Verification items for this drawing (mm, ordinates from the low corner). Round coordinates to 2 decimals unless told otherwise and drop trailing zeros. Loops run counter-clockwise (first coordinate to the right, second up) from the corner with the lowest first, then second, coordinate; pieces in that order, holes last. Notation, with made-up numbers: (-9.75, 46) - (43.25, 46) arc R12 cw to (43.25, 53) - close; hole circle Ø10 at (15.25, 78.5). An arc over 180 degrees is marked (long way). Put each result on its own line as item: value.
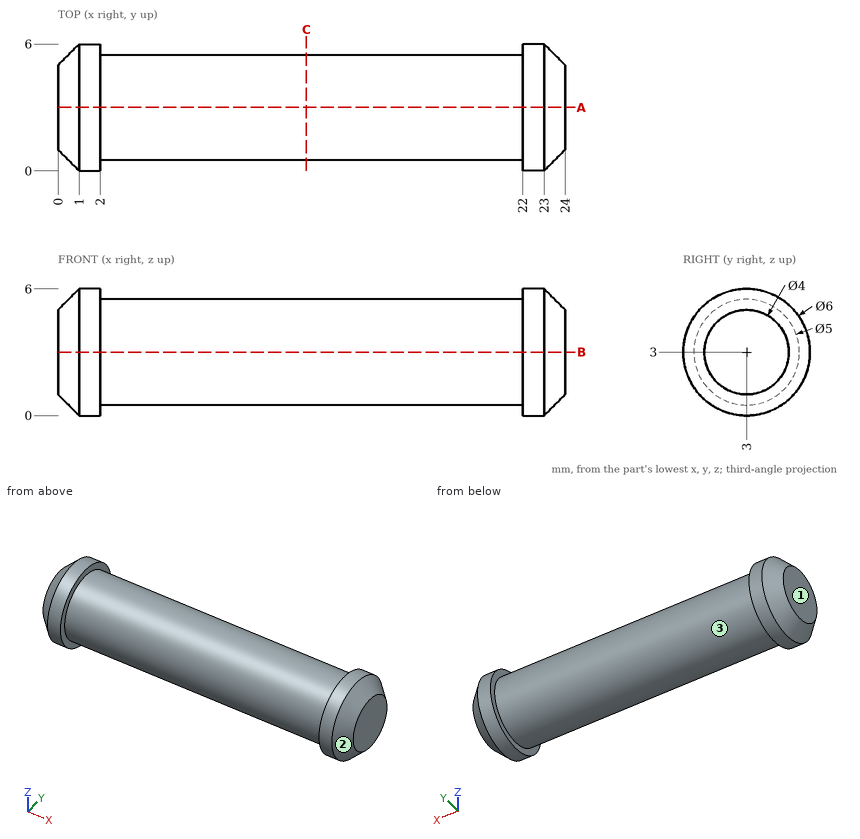
Item 1: Go/stop test with flat-tipped pins: pin 1 (1.5 mm diameter, centred on x = 4, y = 4.5, fed in from +Z); pin 2 (2 mm diameter, centred on x = 10.5, y = 1.5, fed in from -Z). Record where each tip stops, or that it passes through.
Filled sheet:
pin 1: z = 5.38
pin 2: z = 0.55
Item 2: Section check A-A on y = 3. Enter the section's corners in (x, z).
Filled sheet:
outline: (0, 1) - (1, 0) - (2, 0) - (2, 0.5) - (22, 0.5) - (22, 0) - (23, 0) - (24, 1) - (24, 5) - (23, 6) - (22, 6) - (22, 5.5) - (2, 5.5) - (2, 6) - (1, 6) - (0, 5) - close
Item 3: Release check for a two-part mould opening along X. For the marked faces 1, 2 and 3 record: +X half, -X half, draft (parallel to the pull), parting line (faces both ways), or undercut.
Filled sheet:
face 1: -X half
face 2: +X half
face 3: undercut
Item 4: Section check C-C on x = 11.75. Enter the section's corners in (y, z), then the cut area to 3 significant figures.
Filled sheet:
outline: circle Ø5 at (3, 3)
area: 19.6 mm²
Item 5: Thickness scan on line 1 (Z direction, x = 5, y = 1.5); line 2 (X direction, y = 1.35, z = 1.05); line 3 (Y direction, x = 15.75, z = 0.7). Record the ranges inside material, lowest first. Write a range as from..to.
Filled sheet:
line 1: 1..5
line 2: 0.55..2, 22..23.45
line 3: 2.02..3.98
